```python
from build123d import *

# Parameters (mm, degrees)
BOSS_EXTRUDE1_DEPTH = 40
CUT_EXTRUDE1_START  = -16.874456
SKETCH2_R           = 1.5
CUT_EXTRUDE1_DEPTH  = 16.874456
CUT_EXTRUDE3_START  = -17.238427
SKETCH2_4_R         = 2.5
SKETCH2_4_R_2       = 1.5
CUT_EXTRUDE3_DEPTH  = 15.238427
SKETCH3_W           = 30
SKETCH3_H           = 30
SKETCH4_W           = 24
SKETCH4_H           = 24


with BuildPart() as part:
    # Sketch1 → Boss-Extrude1 (new body)
    with BuildSketch(Plane.XY):
        Polygon((50, 18.198511713), (0, 0), (59.816249889, 0), (28.87766783, 85.003055598), (26.058589967, 83.976995168), align=None)
    extrude(amount=BOSS_EXTRUDE1_DEPTH)

    # Sketch2 → Cut-Extrude1 (cut)
    with BuildSketch(Plane.XZ.offset(CUT_EXTRUDE1_START)):
        with Locations((14.954062472, 30)):
            Circle(SKETCH2_R)
        with Locations((44.862187417, 30)):
            Circle(SKETCH2_R)
    cut_extrude1 = extrude(amount=CUT_EXTRUDE1_DEPTH, mode=Mode.SUBTRACT)

    # Sketch2_4 → Cut-Extrude3 (cut)
    with BuildSketch(Plane.XZ.offset(CUT_EXTRUDE3_START)):
        with Locations((14.954062472, 30)):
            Circle(SKETCH2_4_R)
        with Locations((14.954062472, 30)):
            Circle(SKETCH2_4_R_2, mode=Mode.SUBTRACT)
        with Locations((44.862187417, 30)):
            Circle(SKETCH2_4_R)
    cut_extrude3 = extrude(amount=CUT_EXTRUDE3_DEPTH, mode=Mode.SUBTRACT)

    # Mirror1: Cut-Extrude1, Cut-Extrude3 across plane
    add(cut_extrude1.mirror(Plane.XY.offset(20)), mode=Mode.SUBTRACT)
    add(cut_extrude3.mirror(Plane.XY.offset(20)), mode=Mode.SUBTRACT)

    # Sketch3 → Cut-Loft1 section 0
    with BuildSketch(Plane(origin=(50, 18.198511713, 0), x_dir=(0, 0, 1), z_dir=(-0.939692621, -0.342020143, 0))):
        with Locations((20, 50)):
            Rectangle(SKETCH3_W, SKETCH3_H)
    # Sketch4 → Cut-Loft1 section 1
    with BuildSketch(Plane(origin=(52.819077862, 19.224572143, 0), x_dir=(0, 0, -1), z_dir=(0.939692621, 0.342020143, 0))):
        with Locations((-20, 50)):
            Rectangle(SKETCH4_W, SKETCH4_H)
    loft(mode=Mode.SUBTRACT)


solid = part.part
```
Build history of the part. All positions in model axes, mm. A direction names the side the tool comes from. Coordinates: 2 decimals unless noted, no trailing zeros. Order: outer loops, then holes, each group sorted by start corner. A loop starts at its lowest first (then second) coordinate and runs counter-clockwise, first axis right, second up.
Item 1: Drill centre lines: L1, parallel to Y at x = 15.5, z = 32.5; L2, parallel to Y at x = 7.5, z = 22; L3, parallel to X at y = 68, z = 32.5. Where is each one in solid material? Low to high.
Filled in:
L1: y = 0 to 5.64
L2: y = 0 to 2.73
L3: x = 34.53 to 35.07
Item 2: Saw through at A-A on y = 10. List the corners of the cut face in (x, z).
Filled in:
outline: (27.47, 0) - (56.18, 0) - (56.18, 40) - (27.47, 40) - close; hole circle Ø5 at (44.86, 10); hole circle Ø5 at (44.86, 30)
Item 3: Saw through at D-D on y = 48. List the corners of the cut face in (x, z).
Filled in:
outline: (39.15, 0) - (42.35, 0) - (42.35, 40) - (39.15, 40) - close
Item 4: Tool access for faces 4 (the cylindrical face through (46.25, 1.01, 10.57)), 5 (the flat face through (45, 2, 12)), 6 (the flat face through (17, 2, 10)), 7 (the flat face through (27.5, 84.5, 19.7)), 8 (the flat face through (40.52, 44.24, 19.72)): list every direction of +Z, -Z, +X, -X, +Y, -Y with a clear straight run to the whole face (end or side of a thin tool).
Filled in:
face 4: -Y
face 5: none
face 6: +Y
face 7: +Z, -Z, -X, +Y
face 8: +Z, -Z, -X
Item 5: Saw through at B-B on z = 30. State how many separate pieces and enclosed holes the cut face has, then the cut area to 3 significant figures.
Filled in:
separate pieces: 4
enclosed holes: 0
area: 603 mm2
Item 6: Mould opens along Z. For faces 1 (the cylindrical face through (47.247, 9.726, 30.751)), 2 (the flat face through (25.35, 9.227, 19.72)), 3 (the flat face through (41, 14, 0)) say: released by +Z, released by -Z, zero draft, split by the parting line, or undercut.
Filled in:
face 1: undercut
face 2: zero draft
face 3: released by -Z
Item 7: Drop flat-ended pins along their axis: pin 1 Ø4 at (x, z) = (16, 10) entering from +Y; pin 2 Ø1.5 at (x, z) = (14, 30) entering from +Y; pin 3 Ø3 at (y, z) = (49, 14) entering from -X. Give the stop position or say it passes through.
Filled in:
pin 1: stops at y = 6.55
pin 2: stops at y = 2
pin 3: stops at x = 38.24
